from build123d import *

# Parameters (mm, degrees)
BOSS_EXTRUDE1_DEPTH     = 400
SKETCH2_R               = 12.5
CUT_EXTRUDE1_DEPTH      = 1
CUT_EXTRUDE1_DEPTH_BACK = 51
SKETCH4_R               = 3
CUT_EXTRUDE2_DEPTH      = 1
CUT_EXTRUDE2_DEPTH_BACK = 51
SKETCH6_R               = 3
CUT_EXTRUDE3_DEPTH      = 1
CUT_EXTRUDE3_DEPTH_BACK = 51


with BuildPart() as part:
    # Sketch1 → Boss-Extrude1 (new body, symmetric)
    with BuildSketch(Plane.XY):
        Polygon((23.833333333, 42.5), (-26.166666667, 42.5), (-26.166666667, -37.5), (23.833333333, -37.5), (23.833333333, -32.5), (-21.166666667, -32.5), (-21.166666667, 37.5), (23.833333333, 37.5), align=None)
    extrude(amount=BOSS_EXTRUDE1_DEPTH, both=True)

    # Sketch2 → Cut-Extrude1 (cut, two sides)
    with BuildSketch(Plane.ZY.offset(26.166666667)) as cut_extrude1_sk:
        with Locations((-200, 2.5)):
            Circle(SKETCH2_R)
        with Locations((300, 2.5)):
            Circle(SKETCH2_R)
    extrude(amount=CUT_EXTRUDE1_DEPTH, mode=Mode.SUBTRACT)
    extrude(cut_extrude1_sk.sketch, amount=-CUT_EXTRUDE1_DEPTH_BACK, mode=Mode.SUBTRACT)

    # Sketch4 → Cut-Extrude2 (cut, two sides)
    with BuildSketch(Plane.ZY.offset(26.166666667)) as cut_extrude2_sk:
        with Locations((-200.1583434, 27.5)):
            Circle(SKETCH4_R)
        with Locations((-200.1583434, -22.5)):
            Circle(SKETCH4_R)
        with Locations((-175, 3.378177917)):
            Circle(SKETCH4_R)
        with Locations((-224.997353573, 2.863750384)):
            Circle(SKETCH4_R)
    extrude(amount=CUT_EXTRUDE2_DEPTH, mode=Mode.SUBTRACT)
    extrude(cut_extrude2_sk.sketch, amount=-CUT_EXTRUDE2_DEPTH_BACK, mode=Mode.SUBTRACT)

    # Sketch6 → Cut-Extrude3 (cut, two sides)
    with BuildSketch(Plane.ZY.offset(26.166666667)) as cut_extrude3_sk:
        with Locations((299.206047638, 26.660043497)):
            Circle(SKETCH6_R)
        with Locations((325.01367144, 2.494643569)):
            Circle(SKETCH6_R)
        with Locations((300.848271512, -23.312980234)):
            Circle(SKETCH6_R)
        with Locations((275.04064771, 0.852419694)):
            Circle(SKETCH6_R)
    extrude(amount=CUT_EXTRUDE3_DEPTH, mode=Mode.SUBTRACT)
    extrude(cut_extrude3_sk.sketch, amount=-CUT_EXTRUDE3_DEPTH_BACK, mode=Mode.SUBTRACT)


solid = part.part
Geometry check sheet. Reference: the model listing, model coordinates, mm. A direction names the side the tool comes from. Give positions to 0.01 mm unless a question says otherwise; leave off trailing zeros. Loops run counter-clockwise (first coordinate to the right, second up) from the corner with the lowest first, then second, coordinate; pieces in that order, holes last. Notation, with made-up numbers: (26, -11) -> (77, -11) arc R19 cw to (77, 25) -> close; hole circle Ø5 at (35.25, 84). An arc over 180 degrees is marked (long way). Answer in a Markdown table with one row per item. Add a question column.
1) Cross-section at B-B on z = -283. Record the boundary of the cut face in (x, y), and give its area (3 significant figures).
2) Draft check along Y on faces 3 (the face through (-1, 42.5, 6)), 4 (the face through (-24, 6, 312)), 5 (the face through (-26.167, 3, 6)). Enter one of: pulls with the +Y half, pulls with the -Y half, needs draft (parallel to the pull), parting line crosses it, or undercut.
3) Cross-section at A-A on x = -2. Record the boundary of the cut face in (y, z).
4) Set-up check for faces 1 (the face through (2, -32.5, 6)), 2 (the face through (-2, -37.5, 6)): record each of +Z, -Z, +X, -X, +Y, -Y from which the full face is reachable in a straight line by a thin tool's end or side.
5) Material ranges on probe 1 along Y at (x, z) = (-4, 235); probe 2 along X at (y, z) = (-3, 145); probe 3 along Z at (x, y) = (-24, -22), recorded low to high. Write a range as from..to.
6) Gauge pin test, flat ends, axial feed: P1, Ø7, axis at y = 3.38, z = -175, coming from the +X side; P2, Ø9.5, axis at y = 26.66, z = 299.21, coming from the -X side. Record the tip position at first contact, or that the pin passes through.
Outcome:
| question | item | result |
|---|---|---|
| 1 | outline | (-26.17, -37.5) -> (23.83, -37.5) -> (23.83, -32.5) -> (-21.17, -32.5) -> (-21.17, 37.5) -> (23.83, 37.5) -> (23.83, 42.5) -> (-26.17, 42.5) -> close |
| 1 | area | 850 mm^2 |
| 2 | face 3 | pulls with the +Y half |
| 2 | face 4 | undercut |
| 2 | face 5 | needs draft |
| 3 | outline | (-37.5, -400) -> (-32.5, -400) -> (-32.5, 400) -> (-37.5, 400) -> close; (37.5, -400) -> (42.5, -400) -> (42.5, 400) -> (37.5, 400) -> close |
| 4 | face 1 | +Z, -Z, +X |
| 4 | face 2 | +Z, -Z, +X, -X, -Y |
| 5 | probe 1 | y = -37.5..-32.5, 37.5..42.5 |
| 5 | probe 2 | x = -26.17..-21.17 |
| 5 | probe 3 | z = -400..-203.12, -197.2..298.15, 303.55..400 |
| 6 | P1 | stops at x = -21.17 |
| 6 | P2 | stops at x = -26.17 |
